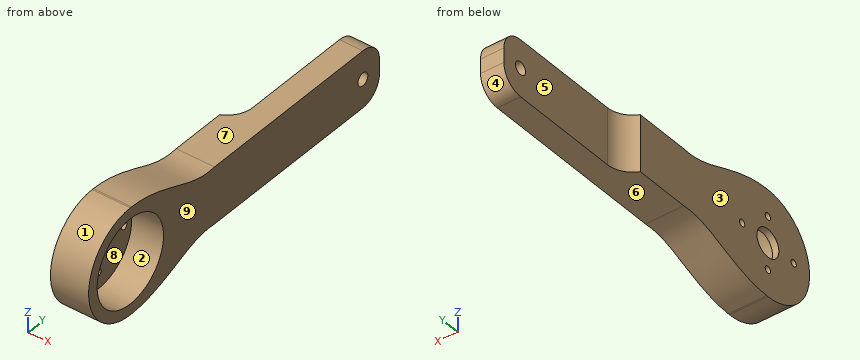
```python
from build123d import *

# Parameters (mm, degrees)
SKETCH1_R               = 10
SKETCH1_R_2             = 0.8
SKETCH1_R_3             = 3.301767793
BOSS_EXTRUDE1_DEPTH     = 1.5
SKETCH2_R               = 10
BOSS_EXTRUDE2_DEPTH     = 9
CUT_EXTRUDE1_DEPTH      = 88.683957995
CUT_EXTRUDE1_DEPTH_BACK = 88.683957995
SKETCH3_R               = 1.5
FILLET1_R               = 5
CUT_EXTRUDE2_DEPTH      = 89.416451723
CUT_EXTRUDE2_DEPTH_BACK = 89.416451723
SKETCH4_W               = 11.042772081
SKETCH4_H               = 46.651109912
FILLET3_R               = 6


with BuildPart() as part:
    # Sketch1 → Boss-Extrude1 (new body)
    with BuildSketch(Plane(origin=(0, 0, 0), x_dir=(0, 0, -1), z_dir=(1, 0, 0))):
        with Locations((2.983378847, 10.826778074)):
            Circle(SKETCH1_R)
        with Locations((2.983378847, 18.576778074)):
            Circle(SKETCH1_R_2, mode=Mode.SUBTRACT)
        with Locations((2.983378847, 3.076778074)):
            Circle(SKETCH1_R_2, mode=Mode.SUBTRACT)
        with Locations((-3.266621153, 10.826778074)):
            Circle(SKETCH1_R_2, mode=Mode.SUBTRACT)
        with Locations((9.233378847, 10.826778074)):
            Circle(SKETCH1_R_2, mode=Mode.SUBTRACT)
        with Locations((2.983378847, 10.826778074)):
            Circle(SKETCH1_R_3, mode=Mode.SUBTRACT)
    extrude(amount=BOSS_EXTRUDE1_DEPTH)

    # Sketch2 → Boss-Extrude2 (add)
    with BuildSketch(Plane.ZY):
        with BuildLine():
            Line((-15.531923741, 85.826778074), (9.565166047, 85.826778074))
            Line((9.565166047, 85.826778074), (9.565166047, 10.826778074))
            ThreePointArc((9.565166047, 10.826778074), (-2.983378847, -1.721766821), (-15.531923741, 10.826778074))
            Line((-15.531923741, 10.826778074), (-15.531923741, 85.826778074))
        make_face()
        with Locations((-2.983378847, 10.826778074)):
            Circle(SKETCH2_R, mode=Mode.SUBTRACT)
    extrude(amount=-BOSS_EXTRUDE2_DEPTH)

    # Sketch3 → Cut-Extrude1 (cut, two sides: drawn at the far end of the back side and taken through both)
    with BuildSketch(Plane(origin=(9, 0, 0), x_dir=(0, 0, -1), z_dir=(1, 0, 0)).offset(-CUT_EXTRUDE1_DEPTH_BACK)):
        with Locations((2.983378847, 80.826778074)):
            Circle(SKETCH3_R)
        with BuildLine():
            Line((-3.709517939, 36.150412664), (-3.709517939, 97.572569437))
            Line((-3.709517939, 97.572569437), (-16.389018159, 97.572569437))
            Line((-16.389018159, 97.572569437), (-16.389018159, 8.14109285))
            Line((-16.389018159, 8.14109285), (-9.565166047, 10.826778074))
            add(Edge.make_bspline(
                [(-9.565166047, 10.826778074), (-9.602791773, 15.116710976), (-7.085897165, 23.501097028), (-3.155123098, 31.470187844), (-3.709517939, 36.150412664)],
                knots=[0, 0, 0, 0, 0.483956382, 1, 1, 1, 1], degree=3))
        make_face()
        with BuildLine():
            Line((22.355775853, 8.14109285), (15.531923741, 10.826778074))
            add(Edge.make_bspline(
                [(15.531923741, 10.826778074), (15.569549467, 15.116710976), (13.052654859, 23.501097028), (9.121880792, 31.470187844), (9.676275633, 36.150412664)],
                knots=[0, 0, 0, 0, 0.483956382, 1, 1, 1, 1], degree=3))
            Line((9.676275633, 36.150412664), (9.676275633, 97.572569437))
            Line((9.676275633, 97.572569437), (22.355775853, 97.572569437))
            Line((22.355775853, 97.572569437), (22.355775853, 8.14109285))
        make_face()
    extrude(amount=CUT_EXTRUDE1_DEPTH + CUT_EXTRUDE1_DEPTH_BACK, mode=Mode.SUBTRACT)

    # Fillet1
    fillet1_edges = [part.edges().sort_by_distance(p)[0] for p in [
        (4.5, 85.826778074, 3.709517939),
        (4.5, 85.826778074, -9.676275633),
    ]]
    fillet(fillet1_edges, radius=FILLET1_R)

    # Sketch4 → Cut-Extrude2 (cut, two sides: drawn at the far end of the back side and taken through both)
    with BuildSketch(Plane(origin=(0, 0, -9.676275633), x_dir=(-1, 0, 0), z_dir=(0, 0, -1)).offset(-CUT_EXTRUDE2_DEPTH_BACK)):
        with Locations((2.021386041, 72.566048538)):
            Rectangle(SKETCH4_W, SKETCH4_H)
    extrude(amount=CUT_EXTRUDE2_DEPTH + CUT_EXTRUDE2_DEPTH_BACK, mode=Mode.SUBTRACT)

    # Fillet3
    # the kernel refuses this fillet: 6 mm, written as the material it adds along each edge
    with BuildSketch(Plane(origin=(3.5, 49.240493582, 3.709517939), x_dir=(-1, 0, 0), z_dir=(0, 0, -1))) as fillet3_piece_1:
        with BuildLine():
            CenterArc((6, 5.454356057), FILLET3_R, 180, 65.375681648)
            Line((0, 5.454356057), (-0.12, 5.454356057))
            Line((-0.12, 5.454356057), (-0.12, 0))
            Line((-0.12, 0), (0, -0.12))
            ThreePointArc((0, -0.12), (1.75, -0.12), (3.45, -0.109087121))
            Line((3.45, -0.109087121), (3.5, 0))
        make_face()
    extrude(amount=13.385793571)


solid = part.part
```
Could you check a few things on this model? Use its own coordinates, in mm. Face numbers are marked on the shaded views. A direction names the side the tool comes from. Round coordinates to 2 decimals unless told otherwise and drop trailing zeros. Loops run counter-clockwise (first coordinate to the right, second up) from the corner with the lowest first, then second, coordinate; pieces in that order, holes last. Notation, with made-up numbers: M -2,4.25 L 33,4.25 A23 cw 33,19.25 Z; hole C 16,-34.75 d2. An arc over 180 degrees is marked long. Answer as CSV lines item,"result".
1) Imagine slicing it at A-A on z = -5.5. List the corners of the cut face in (x, y) for me, and give its area (3 significant figures).
From the geometry:
outline,"M 0,-1.47 L 9,-1.47 L 9,1.15 L 1.5,1.15 L 1.5,8.69 L 0,8.69 Z; M 0,12.96 L 1.5,12.96 L 1.5,20.5 L 9,20.5 L 9,85.76 L 3.5,85.76 L 3.5,54.69 A6 cw 0,49.24 Z"
area,"511 mm^2"
2) For pin 1 Ø2.5 at (y, z) = (10.83, 3.27) entering from +X; pin 2 Ø6.5 at (y, z) = (64.5, -5.5) entering from -X; pin 3 Ø1 at (y, z) = (18.58, -2.98) entering from +X; pin 4 Ø1 at (x, z) = (7, -4) entering from -Y, each with a flat end and sliding along its axis, tell me the tip position at first contact or that it passes through.
From the geometry:
pin 1,"x = 1.5"
pin 2,"x = 3.5"
pin 3,"through"
pin 4,"y = -1.71"
3) Which directions (+Z, -Z, +X, -X, +Y, -Y) give clear straight access to the entire face, cutting with the end or side of a thin tool? Please do the marked faces 5, 6, 7, 8 and 9.
From the geometry:
face 5,"+Z, -Z, -X, +Y"
face 6,"-Z, +X, -X, +Y"
face 7,"+Z, +X, -X, +Y"
face 8,"+X"
face 9,"+Z, -Z, +X, +Y, -Y"
4) Imagine slicing it at D-D on z = 1.25. List the corners of the cut face in (x, y) for me, and give its area (3 significant figures).
From the geometry:
outline,"M 0,-0.99 L 9,-0.99 L 9,1.77 L 1.5,1.77 L 1.5,19.89 L 9,19.89 L 9,85.13 L 3.5,85.13 L 3.5,54.69 A6 cw 0,49.24 Z"
area,"519 mm^2"
5) If I drill on probe 1 along Y at (x, z) = (4.5, -4); probe 2 along X at (y, z) = (75, -8.25); probe 3 along Z at (x, y) = (7.5, 44), over which ranges is the centre line in solid material (lowest first)?
From the geometry:
probe 1,"-1.68 to 0.88, 20.77 to 79.72, 81.93 to 85.83"
probe 2,"3.5 to 9"
probe 3,"-9.68 to 3.71"
6) We'd pull the mould along Y, two halves only. Please class the marked faces 1, 2, 3 and 4: released by +Y, released by -Y, zero draft, split by the parting line, or undercut.
From the geometry:
face 1,"released by -Y"
face 2,"undercut"
face 3,"zero draft"
face 4,"released by +Y"
7) Imagine slicing it at C-C on x = 7. Count the separate pieces of the cut face and the enclosed holes in it, and give its area (3 significant figures).
From the geometry:
separate pieces,"1"
enclosed holes,"2"
area,"1,070 mm^2"
8) Imagine slicing it at B-B on y = 48.5. List the corners of the cut face in (x, z) for me, and give its area (3 significant figures).
From the geometry:
outline,"M 0,-9.68 L 9,-9.68 L 9,3.71 L 0,3.71 Z"
area,"120 mm^2"
